Input: part model. Units: mm. Frame: model coordinates. A direction names the side the tool comes from. Give positions to 0.01 mm unless a question says otherwise; leave off trailing zeros. Loops run counter-clockwise (first coordinate to the right, second up) from the corner with the lowest first, then second, coordinate; pieces in that order, holes last. Notation, with made-up numbers: (-26, 12.25) -> (-10, 12.25) arc R11 ccw to (-10, 29.25) -> close; hole circle Ø7 at (-4, -36.5). An arc over 180 degrees is marked (long way). Use CSV: the item, a comma, the result in double quotes.
Autodesk Fusion 360 part; units mm, degrees
sketch "Sketch3" plane through (0, 0, 0) normal (0, 0, 1) x (1, 0, 0)
  circle A0 centre (26.3947, 0) radius 8
  circle A1 centre (26.3947, 0) radius 11
  dimension "d13" = 16
  dimension "d14" = 22
extrude "Extrude4" add sketch "Sketch3" along normal blind 10
sketch "Sketch4" plane through (0, 0, 10) normal (0, 0, 1) x (-1, 0, 0)
  circle A0 centre (-26.3947, 0) radius 8
  circle A1 centre (-26.3947, 0) radius 11
  circle A2 centre (-26.3947, 0) radius 13
  circle A3 centre (-26.3947, 0) radius 8
  dimension "d17" = 26
extrude "Extrude5" add sketch "Sketch4" against normal blind 1.5 contours A2
sketch "Sketch5" plane through (0, 0, 0) normal (0, 0, -1) x (1, 0, 0)
  circle A0 centre (26.3947, 0) radius 8
  circle A1 centre (26.3947, 0) radius 11
  circle A2 centre (26.3947, 0) radius 12.5
  dimension "d20" = 25
extrude "Extrude6" add sketch "Sketch5" against normal blind 1.5 contours A2
fillet "Fillet2" radius 1 1 edges at (16.1391, 3.9778, 8.5)
sketch "Sketch6" plane through (0, 0, 0) normal (0, 0, -1) x (1, 0, 0)
  circle A0 centre (26.3947, 0) radius 12.5
  circle A1 centre (26.3947, 0) radius 8
  circle A2 centre (26.3947, 0) radius 7
  dimension "d25" = 14
extrude "Extrude7" add sketch "Sketch6" against normal blind 5.3 contours A1
1) Contact query for flat-ended pins moving along their axis: pin 1 (1.5 mm diameter, centred on x = 21.5, z = 1.5, fed in from -Y); pin 2 (1.5 mm diameter, centred on x = 21.5, z = 4, fed in from +Y); pin 3 (2 mm diameter, centred on y = -1.5, z = 3.5, fed in from +X). Output: stop coordinate, or through.
From the geometry:
pin 1,"stops at y = -11.79"
pin 2,"stops at y = 10.19"
pin 3,"stops at x = 37.38"
2) Section query A-A (y = 0). Return loops of the section in (x, z).
From the geometry:
outline,"(13.39, 8.5) -> (14.39, 8.5) arc R1 cw to (15.39, 7.5) -> (15.39, 1.5) -> (13.89, 1.5) -> (13.89, 0) -> (19.39, 0) -> (19.39, 5.3) -> (18.39, 5.3) -> (18.39, 10) -> (13.39, 10) -> close; (33.39, 0) -> (38.89, 0) -> (38.89, 1.5) -> (37.39, 1.5) -> (37.39, 7.5) arc R1 cw to (38.39, 8.5) -> (39.39, 8.5) -> (39.39, 10) -> (34.39, 10) -> (34.39, 5.3) -> (33.39, 5.3) -> close"
3) Section query C-C (z = 4). Return loops of the section in (x, y).
From the geometry:
outline,"circle Ø22 at (26.39, 0); hole circle Ø14 at (26.39, 0)"
4) Ray query, line 1 (Y direction, x = 26.25, z = 3.5); line 2 (X direction, y = 0, z = 6.65); line 3 (Y direction, x = 29.75, z = 3.25). Return the intervals inside material, ascending.
From the geometry:
line 1,"y = -11 to -7, 7 to 11"
line 2,"x = 15.39 to 18.39, 34.39 to 37.39"
line 3,"y = -10.48 to -6.14, 6.14 to 10.48"
5) Section query B-B (z = 9.25). Return loops of the section in (x, y), then the cut area to 3 significant figures.
From the geometry:
outline,"circle Ø26 at (26.39, 0); hole circle Ø16 at (26.39, 0)"
area,"330 mm^2"
6) Mould query, pull axis X, two halves, no side actions, for faces 1 (the flat face through (32, 5, 5.3)), 2 (the flat face through (33, 9, 1.5)), 3 (the cylindrical face through (38.32, -3.75, 0.74)). Classes: pulls with the +X half, pulls with the -X half, needs draft (parallel to the pull), parting line crosses it, or undercut.
From the geometry:
face 1,"undercut"
face 2,"needs draft"
face 3,"parting line crosses it"
7) Reachability of faces 4 (the flat face through (32, 5, 0)), 5 (the cylindrical face through (24.66, 7.81, 7.62)), 6 (the cylindrical face through (15.405, -0.484, 4.458)) from +Z, -Z, +X, -X, +Y, -Y: full face, straight path, thin tool, end or side. Return the list, or none.
From the geometry:
face 4,"-Z, +X, -X, +Y, -Y"
face 5,"+Z"
face 6,"none"
